Source: CAD feature listing. Evaluate the final solid. Frame: model axes, mm. Face numbers are marked on the shaded views. A direction names the side the tool comes from. Coordinates: 2 decimals unless noted, no trailing zeros. Order: outer loops, then holes, each group sorted by start corner. A loop starts at its lowest first (then second) coordinate and runs counter-clockwise, first axis right, second up.
```python
from build123d import *
from build123d.topology import SkipClean

# Parameters (mm, degrees)
SKETCH1_R           = 1.6
BOSS_EXTRUDE1_DEPTH = 20
SKETCH3_R           = 2.6
BOSS_EXTRUDE2_DEPTH = 13


with BuildPart() as part:
    # Sketch1 → Boss-Extrude1 (new body)
    with BuildSketch(Plane(origin=(0, 0, 0), x_dir=(1, 0, 0), z_dir=(0, 1, 0))):
        with BuildLine():
            Line((165, -8), (165, 0))
            Line((165, 0), (84, 0))
            Line((84, 0), (84, -4))
            Line((84, -4), (149.183346174, -4))
            ThreePointArc((149.183346174, -4), (153.020959068, -5.387763311), (155.08333917, -8.909090909))
            ThreePointArc((155.08333917, -8.909090909), (160.456451448, -12.979121617), (165, -8))
        make_face()
        with Locations(Location((160, -8, 0), (0, 0, 270))):
            Circle(SKETCH1_R, mode=Mode.SUBTRACT)
    extrude(amount=BOSS_EXTRUDE1_DEPTH)


with BuildPart() as body_2:
    # Sketch3 → Boss-Extrude2 (new, through all)
    with BuildSketch(Plane.XY):
        with BuildLine():
            Line((122, 0), (165, 0))
            Line((165, 0), (165, 9))
            Line((165, 9), (153.284271247, 9))
            ThreePointArc((153.284271247, 9), (149.457436924, 9.761204675), (146.213203436, 11.928932188))
            Line((146.213203436, 11.928932188), (141.071067812, 17.071067812))
            ThreePointArc((141.071067812, 17.071067812), (137.826834324, 19.238795325), (134, 20))
            Line((134, 20), (84, 20))
            Line((84, 20), (84, 12.6))
            ThreePointArc((84, 12.6), (85.838477631, 11.838477631), (86.6, 10))
            ThreePointArc((86.6, 10), (85.838477631, 8.161522369), (84, 7.4))
            Line((84, 7.4), (84, 0))
            Line((84, 0), (114, 0))
            ThreePointArc((114, 0), (118, 4), (122, 0))
        make_face()
        with Locations(Location((134, 10, 0), (0, 0, 180))):
            Circle(SKETCH3_R, mode=Mode.SUBTRACT)
    extrude(amount=BOSS_EXTRUDE2_DEPTH)

    # Intersect1: read off the stored shape, not the designer's step
    # Intersect1: intersect part
    add(part.part, mode=Mode.INTERSECT)

    # Mirror1: body 2 across face


with BuildPart() as body_2_1:
    with SkipClean():  # the faces are left unmerged after this step: merging them gives an invalid solid
        add(body_2.part)
        add(body_2.part.mirror(Plane(origin=(84, 16.3, 2), x_dir=(0, 0, 1), z_dir=(-1, 0, 0))))


solid = body_2_1.part
```
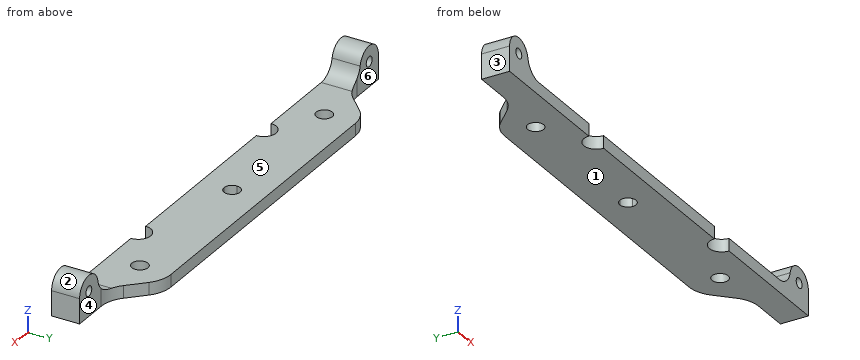
Q1. Pull-direction query (X, two-part tool) for the marked faces 1, 2 and 3; classes: pulls with the +X half, pulls with the -X half, needs draft (parallel to the pull), parting line crosses it, or undercut.
Solutions:
face 1: needs draft
face 2: undercut
face 3: pulls with the -X half
Q2. Section query A-A on x = 8. Output: boundary loops of the cut face in (y, z), plus the area to 3 significant figures.
Solutions:
outline: (0, 0) - (9, 0) - (9, 6.4) - (0, 6.4) - close; (0, 9.6) - (9, 9.6) - (9, 13) - (0, 13) - close
area: 88.2 mm2
Q3. Section query B-B on x = 50. Output: boundary loops of the cut face in (y, z).
Solutions:
outline: (4, 0) - (20, 0) - (20, 4) - (4, 4) - close
Q4. Pin query (flat end, axial travel): P1, Ø2, axis at x = 101, y = 6.5, coming from the +Z side; P2, Ø3.5, axis at x = 159.5, z = 6, coming from the +Y side. Return the tip coordinate at first contact, or that it passes through.
Solutions:
P1: stops at z = 4
P2: stops at y = 9
Q5. Set-up query: the marked faces 4, 5 and 6. Return all of +Z, -Z, +X, -X, +Y, -Y with unobstructed straight access to the full face (end or side cutting, diameter ignored); none if empty.
Solutions:
face 4: +Z, -Z, +X, +Y
face 5: +Z, +Y, -Y
face 6: +Z, -Z, -X, +Y
Q6. Material intervals for line 1 along X through (y, z) = (2.75, 8); line 2 along Y through (x, z) = (134, 1.5); line 3 along Z through (x, y) = (160, 2), sorted ascending.
Solutions:
line 1: x = 3 to 6.4, 9.6 to 13.16, 154.84 to 158.4, 161.6 to 165
line 2: y = 0 to 7.4, 12.6 to 20
line 3: z = 0 to 6.4, 9.6 to 13
